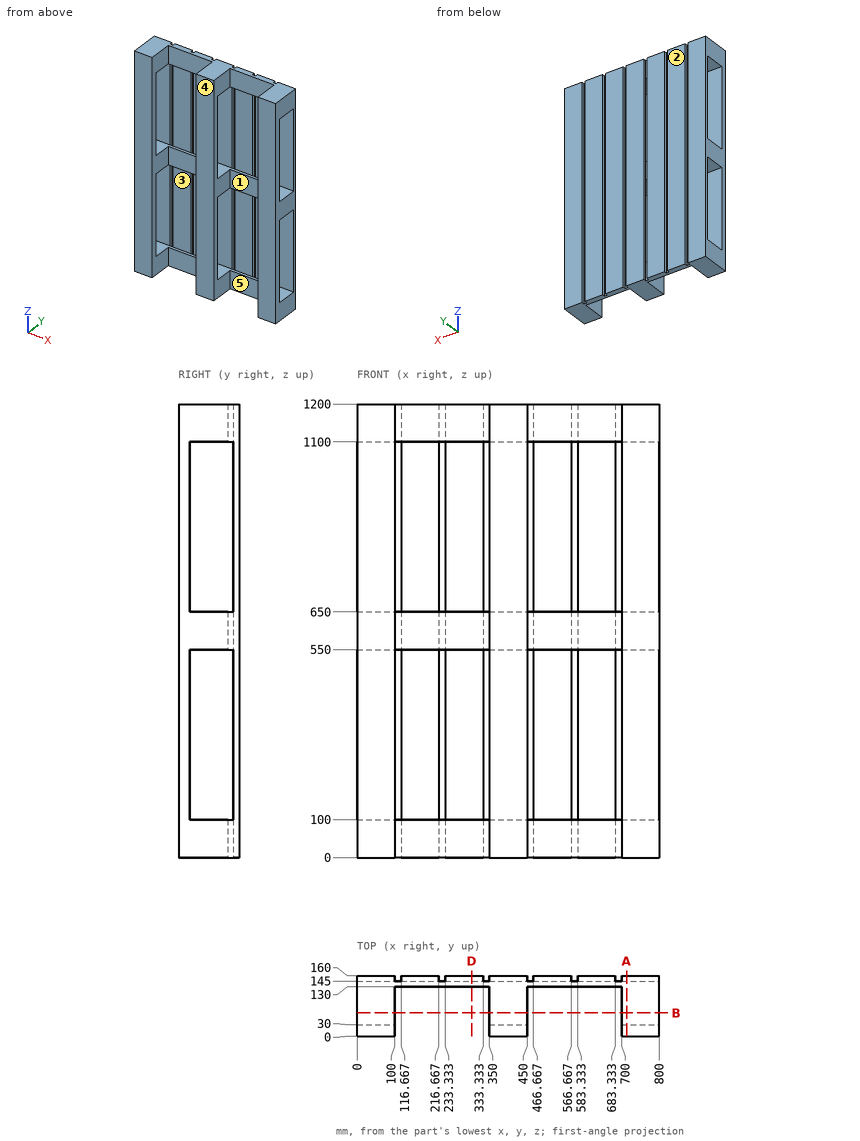
Answer from the drawing. Dimensions are ordinates in mm from the lowest x, y and z of the part. A direction names the side the tool comes from. Give positions to 0.01 mm unless a question says otherwise; leave off trailing zeros. Write each loop counter-clockwise with the first axis right and the second up, starting at its lowest first coordinate (ties: lowest second). Pieces come first, ordered by that corner, then holes. Notation, with made-up numbers: (-36, -36) - (-7, -36) arc R28 cw to (-7, -11) - close; hole circle Ø9 at (2.5, 37). An arc over 180 degrees is marked (long way). One line per item, written item: value. Start each with the question number.
1. For a pull along X with two mould halves and no side action, classify the marked faces 1 and 2 as +X half, -X half, draft (parallel to the pull), parting line (faces both ways), or undercut.
2. Find section D-D (x = 303). Write down the section's boundary in (y, z).
3. For the marked faces 3, 4 and 5, determine the directions among +Z, -Z, +X, -X, +Y, -Y from which every point of the face is accessible in a straight line to the end or side of a thin tool.
4. Consider probe 1 along Z at (x, y) = (732.5, 116.5); probe 2 along X at (y, z) = (19.5, 975.5); probe 3 along Y at (x, z) = (446, 483.5). Determine where each line is inside the solid, lowest interval first.
5. Find section A-A (x = 713). Write down the section's boundary in (y, z), then the cut area to 3 significant figures.
6. Find section B-B (y = 61). State how many separate pieces and enclosed holes the cut face has, then the cut area to 3 significant figures.
7. Given pin 1 (16.5 mm diameter, centred on y = 156, z = 567.5, fed in from -X); pin 2 (13.5 mm diameter, centred on x = 574, z = 593, fed in from +Y), each flat-ended and moving along its own axis, determine where each tip first touches the part or whether it passes through.
Geometry results:
1. face 1: undercut
1. face 2: draft
2. outline: (130, 0) - (160, 0) - (160, 1200) - (130, 1200) - (130, 1100) - (145, 1100) - (145, 650) - (130, 650) - (130, 550) - (145, 550) - (145, 100) - (130, 100) - close
3. face 3: +X, -X, -Y
3. face 4: +Z, -Z, +X, -X, -Y
3. face 5: +Z, -Z, -Y
4. probe 1: 0 to 100, 550 to 650, 1100 to 1200
4. probe 2: 0 to 100, 350 to 450, 700 to 800
4. probe 3: 0 to 30, 145 to 160
5. outline: (0, 0) - (160, 0) - (160, 1200) - (0, 1200) - close; hole (30, 100) - (145, 100) - (145, 550) - (30, 550) - close; hole (30, 650) - (145, 650) - (145, 1100) - (30, 1100) - close
5. area: 88,500 mm2
6. separate pieces: 9
6. enclosed holes: 0
6. area: 90,000 mm2
7. pin 1: x = 0
7. pin 2: y = 145
